Can you work these out from the model? Positions are in its coordinate system, mm. Face numbers are marked on the shaded views. A direction names the side the tool comes from. Coordinates: 2 decimals unless noted, no trailing zeros. Loops run counter-clockwise (first coordinate to the right, second up) from the corner with the lowest first, then second, coordinate; pieces in that order, holes last.
```python
from build123d import *

# Parameters (mm, degrees)
SKETCH1_R           = 12.5
BOSS_EXTRUDE1_DEPTH = 5.1


with BuildPart() as part:
    # Sketch1 → Boss-Extrude1 (new body)
    with BuildSketch(Plane.XY):
        with BuildLine():
            Line((0, 0), (-4.9, 0))
            Line((-4.9, 0), (-4.9, -5.1))
            Line((-4.9, -5.1), (-10, -5.1))
            Line((-10, -5.1), (-10, 0))
            Line((-10, 0), (-30, 0))
            Line((-30, 0), (-30, -5.1))
            Line((-30, -5.1), (-35.1, -5.1))
            Line((-35.1, -5.1), (-35.1, 0))
            Line((-35.1, 0), (-40, 0))
            Line((-40, 0), (-40, 14.5))
            ThreePointArc((-40, 14.5), (-20, 34.5), (0, 14.5))
            Line((0, 14.5), (0, 0))
        make_face()
        with Locations((-20, 14.5)):
            Circle(SKETCH1_R, mode=Mode.SUBTRACT)
    extrude(amount=BOSS_EXTRUDE1_DEPTH)


solid = part.part
```
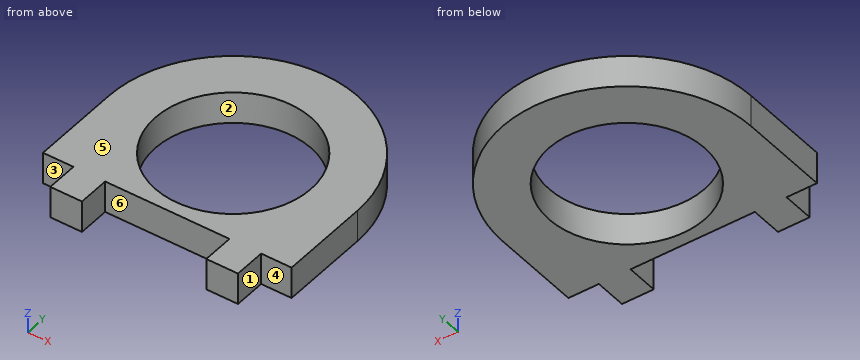
Item 1: Suppose I cut it at A-A, the plane y = 17.5. Please give me the cut outline in (x, z), plus the area to 3 significant figures.
Results are:
outline: (-39.77, 0) - (-32.13, 0) - (-32.13, 5.1) - (-39.77, 5.1) - close; (-7.87, 0) - (-0.23, 0) - (-0.23, 5.1) - (-7.87, 5.1) - close
area: 77.9 mm2
Item 2: On a 3-axis mill with a long thin cutter (end or side, diameter ignored), from which of +Z, -Z, +X, -X, +Y, -Y can I reach the whole of each face in a straight line? I mean the marked faces 4, 5 and 6. Say none if no direction works.
Results are:
face 4: +Z, -Z, +X, -Y
face 5: +Z, +X, -X, +Y, -Y
face 6: +Z, -Z, -Y
Item 3: We'd pull the mould along X, two halves only. Please class the marked faces 1, 2 and 3: +X half, -X half, draft (parallel to the pull), parting line (faces both ways), or undercut.
Results are:
face 1: +X half
face 2: undercut
face 3: draft
Item 4: Suppose I cut it at B-B, the plane x = -20. Please give me the cut outline in (y, z), plus the area to 4 significant figures.
Results are:
outline: (0, 0) - (2, 0) - (2, 5.1) - (0, 5.1) - close; (27, 0) - (34.5, 0) - (34.5, 5.1) - (27, 5.1) - close
area: 48.45 mm2
Item 5: I'm going to push flat-ended pins straight in: P1, Ø1.5, axis at y = -3.5, z = 3, coming from the -X side; P2, Ø2, axis at y = 13.5, z = 2.5, coming from the +X side; P3, Ø22.5, axis at x = -20, y = 14.5, coming from the -Z side; P4, Ø2.5, axis at y = -1.5, z = 3.5, coming from the +X side. Where does each tip first touch, or does it pass through?
Results are:
P1: stops at x = -35.1
P2: stops at x = 0
P3: passes through
P4: stops at x = -4.9
Item 6: Suppose I cut it at C-C, the plane z = 0.75. Please give me the cut outline in (x, y).
Results are:
outline: (-40, 0) - (-35.1, 0) - (-35.1, -5.1) - (-30, -5.1) - (-30, 0) - (-10, 0) - (-10, -5.1) - (-4.9, -5.1) - (-4.9, 0) - (0, 0) - (0, 14.5) arc R20 ccw to (-40, 14.5) - close; hole circle Ø25 at (-20, 14.5)
Item 7: I need wall thicknesses on line 1 along Y through (x, z) = (-20, 2.95); line 2 along X through (y, z) = (-0.5, 1.55); line 3 along X through (y, z) = (14, 3.7). Which ranges of each line are inside material? Lowest first, please.
Results are:
line 1: y = 0 to 2, 27 to 34.5
line 2: x = -35.1 to -30, -10 to -4.9
line 3: x = -40 to -32.49, -7.51 to 0
Item 8: Suppose I cut it at D-D, the plane x = -36. Please give me the cut outline in (y, z).
Results are:
outline: (0, 0) - (26.5, 0) - (26.5, 5.1) - (0, 5.1) - close
